Solid Edge part; units mm, degrees
sketch "Sketch1" plane through (0, 0, 0) normal (0, -1, 0) x (1, 0, 0)
  line L0 (-136.525, 48.4187) -> (135.763, 48.4187)
  line L1 (135.763, 48.4187) -> (135.763, -48.4187)
  line L2 (135.763, -48.4187) -> (-136.525, -48.4188)
  line L3 (-136.525, -48.4188) -> (-136.525, 48.4187)
  dimension "D1" = 136.525
  dimension "D2" = 136.525
extrude "Protrusion1" add sketch "Sketch1" along normal mid plane 241.3
sketch "Sketch2" plane through (0, 0, 0) normal (1, 0, 0) x (0, 1, 0)
  line L0 (101.6, -48.4187) -> (-101.6, -48.4188)
  line L1 (-101.6, -48.4188) -> (-101.6, 48.4187)
  line L2 (-101.6, 48.4187) -> (101.6, 48.4188)
  line L3 (101.6, 48.4188) -> (101.6, -48.4187)
extrude "Cutout1" cut sketch "Sketch2" along normal up to next and the other way up to next
sketch "Sketch3" plane through (6.4194, -101.6, 0) normal (0, 1, 0) x (-1, 0, 0)
  line L0 (138.1819, -43.6563) -> (15.9444, -43.6563)
  line L1 (15.9444, -48.4188) -> (15.9444, -43.6563)
  line L2 (15.9444, -48.4188) -> (142.9444, -48.4188)
  line L3 (142.9444, -48.4188) -> (142.9444, 48.4187)
  line L4 (142.9444, 48.4187) -> (15.9444, 48.4187)
  line L5 (15.9444, 43.6562) -> (15.9444, 48.4187)
  line L6 (15.9444, 43.6562) -> (138.1819, 43.6562)
  line L7 (138.1819, 43.6562) -> (138.1819, -43.6563)
extrude "ExtrudedCutout_2" cut sketch "Sketch3" against normal blind 12.7
mirror "Mirror1" about plane through (0, 0, 0) normal (0, 1, 0) of "ExtrudedCutout_2"
sketch "Sketch4" plane through (21.4313, 101.6, 12.7) normal (0, -1, 0) x (1, 0, 0)
  circle A0 centre (-107.1563, 0) radius 14.2875
extrude "ExtrudedCutout_3" cut sketch "Sketch4" against normal blind 7.62
mirror "Mirror2" about plane through (0, 0, 0) normal (0, -1, 0) of "ExtrudedCutout_3"
sketch "Sketch5" plane through (6.4194, 0, 0) normal (0, -1, 0) x (1, 0, 0)
  line L0 (-15.9444, -43.6563) -> (3.1056, -43.6563)
  line L1 (3.1056, -43.6563) -> (3.1056, 48.4188)
  line L2 (3.1056, 48.4188) -> (-15.9444, 48.4188)
  line L3 (-15.9444, 48.4188) -> (-15.9444, -43.6563)
  dimension "D1" = 15.9444
extrude "Protrusion2" add sketch "Sketch5" along normal up to next and the other way up to next
sketch "Sketch6" plane through (0, 0, 0) normal (1, 0, 0) x (0, 1, 0)
  line L0 (31.75, -29.3687) -> (-31.75, -29.3688)
  line L1 (-31.75, -29.3688) -> (-31.75, 34.1312)
  line L2 (-31.75, 34.1313) -> (31.75, 34.1313)
  line L3 (31.75, 34.1313) -> (31.75, -29.3687)
  circle A0 centre (-35, 37.3813) radius 1.9984
  circle A1 centre (-35, -32.6187) radius 1.7985
  circle A2 centre (35, 37.3813) radius 1.7985
  circle A3 centre (35, -32.6187) radius 1.7985
  dimension "D1" = 31.75
  dimension "D2" = 31.75
extrude "Cutout2" cut sketch "Sketch6" along normal up to next and the other way up to next
sketch "Sketch7" plane through (-9.525, 0, 3.175) normal (-1, 0, 0) x (0, -1, 0)
  circle A0 centre (-57.15, 3.175) radius 4.7625
  circle A1 centre (63.5, 3.175) radius 4.7625
extrude "Cutout3" cut sketch "Sketch7" against normal up to next
sketch "Sketch8" plane through (-136.525, 117.475, 0) normal (-1, 0, 0) x (0, 0, 1)
  line L0 (-43.6563, -3.175) -> (-48.4188, -3.175)
  line L1 (-48.4188, -3.175) -> (-48.4188, -15.875)
  line L2 (-48.4188, -15.875) -> (-43.6563, -15.875)
  line L3 (-43.6563, -15.875) -> (-43.6563, -3.175)
extrude "Cutout4" cut sketch "Sketch8" against normal up to next
mirror "Mirror3" about plane through (0, 0, 0) normal (0, -1, 0) of "Cutout4"
Source: CAD feature listing. Evaluate the final solid. Frame: model axes, mm. A direction names the side the tool comes from. Coordinates: 2 decimals unless noted, no trailing zeros. Loops run counter-clockwise (first coordinate to the right, second up) from the corner with the lowest first, then second, coordinate; pieces in that order, holes last. Notation, with made-up numbers: (63.5, -31.5) -> (120.5, -31.5) arc R16 ccw to (120.5, -23.5) -> close; hole circle Ø3 at (41.25, 62). An arc over 180 degrees is marked (long way). One line per item, written item: value. Start each with the question number.
Q1. Set-up query: faces 1 (the face through (-71, 108, 43.656)), 2 (the face through (-100, -105.4, 12.1)), 3 (the face through (72, 101.6, 3)), 4 (the face through (1, 26, -43.656)). Return all of +Z, -Z, +X, -X, +Y, -Y with unobstructed straight access to the full face (end or side cutting, diameter ignored); none if empty.
Q2. Contact query for flat-ended pins moving along their axis: P1, Ø14, axis at y = 110.5, z = 17.5, coming from the -X side (3 decimals); P2, Ø15, axis at x = -3, y = -7.5, coming from the -Z side; P3, Ø3, axis at y = 89.5, z = -1, coming from the -X side (3 decimals); P4, Ø7.5, axis at y = 57.15, z = 6.35, coming from the -X side. Output: stop coordinate, or through.
Q3. Section query D-D, the plane x = 0. Give the number of separate pieces and of enclosed holes in the cut face, and give its area (3 significant figures).
Q4. Mould query, pull axis Y, two halves, no side actions, for faces 5 (the face through (135.763, 111, 1)), 6 (the face through (-20, -114.3, -47)), 7 (the face through (2, -120.65, -1)). Classes: pulls with the +Y half, pulls with the -Y half, needs draft (parallel to the pull), parting line crosses it, or undercut.
Q5. Line query: line 1 along Z through (x, y) = (-4, -35); line 2 along Z through (x, y) = (2, -63.5); line 3 along Z through (x, y) = (-1.25, 35). Output: solid intervals per line, ascending.
Q6. Section query C-C, the plane y = 4. Return the cut outline in (x, z) (3 decimals).
Q7. Section query B-B, the plane x = -113.5. Return the cut outline in (y, z).
Results:
1. face 1: +Z, -X
1. face 2: none
1. face 3: +Z, -Z, +X
1. face 4: -Z, +X, -X
2. P1: x = -136.525
2. P2: z = -43.66
2. P3: x = -9.525
2. P4: through
3. separate pieces: 1
3. enclosed holes: 7
3. area: 18,100 mm^2
4. face 5: needs draft
4. face 6: undercut
4. face 7: pulls with the -Y half
5. line 1: -43.66 to -34.42, -30.82 to 35.38, 39.38 to 48.42
5. line 2: -43.66 to 1.59, 11.11 to 48.42
5. line 3: -43.66 to -34.42, -30.82 to 35.58, 39.18 to 48.42
6. outline: (-9.525, -43.656) -> (9.525, -43.656) -> (9.525, -29.369) -> (-9.525, -29.369) -> close; (-9.525, 34.131) -> (9.525, 34.131) -> (9.525, 48.419) -> (-9.525, 48.419) -> close
7. outline: (-120.65, -48.42) -> (-114.3, -48.42) -> (-114.3, -43.66) -> (-101.6, -43.66) -> (-101.6, 43.66) -> (-114.3, 43.66) -> (-114.3, 48.42) -> (-120.65, 48.42) -> close; (101.6, -43.66) -> (114.3, -43.66) -> (114.3, -48.42) -> (120.65, -48.42) -> (120.65, 48.42) -> (114.3, 48.42) -> (114.3, 43.66) -> (101.6, 43.66) -> close
